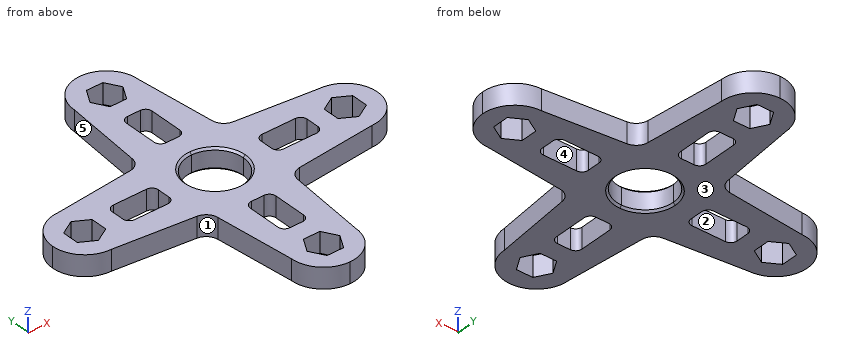
from build123d import *

# Parameters (mm, degrees)
F1_DEPTH = 8
F3_COUNT = 4
F4_R     = 5
F5_SIZE  = 0.762


with BuildPart() as f1:
    # F0 (on Top) → F1 (new body)
    with BuildSketch(Plane.XY):
        with BuildLine():
            ThreePointArc((0, 63.3), (-8.8388347648, 59.6388347648), (-12.5, 50.8))
            Line((-12.5, 50.8), (-6.4172713361, 50.8))
            Line((-6.4172713361, 50.8), (-3.208635668, 56.35752))
            Line((-3.208635668, 56.35752), (0, 56.35752))
            Line((0, 56.35752), (0, 63.3))
        make_face()
        with BuildLine():
            Line((6.4172713361, 50.8), (12.5, 50.8))
            ThreePointArc((12.5, 50.8), (8.8388347648, 59.6388347648), (0, 63.3))
            Line((0, 63.3), (0, 56.35752))
            Line((0, 56.35752), (3.208635668, 56.35752))
            Line((3.208635668, 56.35752), (6.4172713361, 50.8))
        make_face()
        with BuildLine():
            ThreePointArc((0, 38.3), (8.8388347648, 41.9611652352), (12.5, 50.8))
            Line((12.5, 50.8), (6.4172713361, 50.8))
            Line((6.4172713361, 50.8), (3.208635668, 45.24248))
            Line((3.208635668, 45.24248), (0, 45.24248))
            Line((0, 45.24248), (0, 38.3))
        make_face()
        with BuildLine():
            Line((-6.4172713361, 50.8), (-12.5, 50.8))
            ThreePointArc((-12.5, 50.8), (-8.8388347648, 41.9611652352), (0, 38.3))
            Line((0, 38.3), (0, 45.24248))
            Line((0, 45.24248), (-3.208635668, 45.24248))
            Line((-3.208635668, 45.24248), (-6.4172713361, 50.8))
        make_face()
        with BuildLine():
            ThreePointArc((-17.4128947138, 1.7438743322), (-11.7416395615, 12.9762822259), (0, 17.5))
            Line((0, 17.5), (0, 20))
            Line((0, 20), (-2.5, 20))
            ThreePointArc((-2.5, 20), (-4.267766953, 20.732233047), (-5, 22.5))
            Line((-5, 22.5), (-5, 35.5))
            ThreePointArc((-5, 35.5), (-4.267766953, 37.267766953), (-2.5, 38))
            Line((-2.5, 38), (0, 38))
            Line((0, 38), (0, 38.3))
            ThreePointArc((0, 38.3), (-8.8388347648, 41.9611652352), (-12.5, 50.8))
            Line((-12.5, 50.8), (-17.4128947138, 1.7438743322))
        make_face()
        with BuildLine():
            Line((0, 20), (0, 17.5))
            ThreePointArc((0, 17.5), (11.7416395615, 12.9762822259), (17.4128947138, 1.7438743322))
            Line((17.4128947138, 1.7438743322), (12.5, 50.8))
            ThreePointArc((12.5, 50.8), (8.8388347648, 41.9611652352), (0, 38.3))
            Line((0, 38.3), (0, 38))
            Line((0, 38), (2.5, 38))
            ThreePointArc((2.5, 38), (4.267766953, 37.267766953), (5, 35.5))
            Line((5, 35.5), (5, 22.5))
            ThreePointArc((5, 22.5), (4.267766953, 20.732233047), (2.5, 20))
            Line((2.5, 20), (0, 20))
        make_face()
        with BuildLine():
            ThreePointArc((17.4128947138, 1.7438743322), (11.7416395615, 12.9762822259), (0, 17.5))
            ThreePointArc((0, 17.5), (-11.7416395615, 12.9762822259), (-17.4128947138, 1.7438743322))
            ThreePointArc((-17.4128947138, 1.7438743322), (-0.8730242003, -17.4782101128), (17.5, 0))
            ThreePointArc((17.5, 0), (17.4782101128, 0.8730242003), (17.4128947138, 1.7438743322))
        make_face()
        with BuildLine():
            ThreePointArc((0, 11.025), (7.7958522626, 7.7958522626), (11.025, 0))
            ThreePointArc((11.025, 0), (-7.7958522626, -7.7958522626), (0, 11.025))
        make_face(mode=Mode.SUBTRACT)
    extrude(amount=F1_DEPTH)

    # F3: F1 ×4 about axis
    f3_axis = Axis((0, 0, 24.1194125265), (0, 0, 1))


with BuildPart() as f1_1:
    add(f1.part)
    for i in range(1, F3_COUNT):
        add(f1.part.rotate(f3_axis, i * 360 / F3_COUNT))

    # F4
    f4_edges = [f1_1.edges().sort_by_distance(p)[0] for p in [
        (15.986516, 15.986516, 4),
        (-15.986516, 15.986516, 4),
        (-15.986516, -15.986516, 4),
        (15.986516, -15.986516, 4),
    ]]
    fillet(f4_edges, radius=F4_R)

    # F5
    f5_edges = [f1_1.edges().sort_by_distance(p)[0] for p in [
        (0, -11.025, 8),
        (0, -11.025, 0),
    ]]
    chamfer(f5_edges, length=F5_SIZE)


solid = f1_1.part
Part model, mm, in its own coordinate system. Face numbers are marked on the shaded views. A direction names the side the tool comes from. Give positions to 0.01 mm unless a question says otherwise; leave off trailing zeros. Loops run counter-clockwise (first coordinate to the right, second up) from the corner with the lowest first, then second, coordinate; pieces in that order, holes last. Notation, with made-up numbers: (49, 8.25) -> (102, 8.25) arc R33 ccw to (102, 43.25) -> close; hole circle Ø4 at (30, 37.25). An arc over 180 degrees is marked (long way). Write each question's results on one line, items separated by ' | '. Start each with the question number.
Q1. Band-saw the part on B-B on z = 5.25. Count the separate pieces of the cut face and the enclosed holes in it, plus the area to 3 significant figures.
Q2. Band-saw the part on A-A on x = -28. List the corners of the cut face in (y, z), plus the area to 3 significant figures.
Q3. Pull direction X, two halves, no side cores. Call the marked faces 1, 2 and 3: +X half, -X half, draft (parallel to the pull), parting line (faces both ways), or undercut.
Q4. Pin check, flat tips, straight feed: P1, Ø4, axis at x = 44.5, z = 4, coming from the +Y side; P2, Ø4, axis at y = 29, z = 4.5, coming from the -X side; P3, Ø4, axis at x = 28, z = 5, coming from the -Y side. Stop position of each tip, or through.
Q5. Wall check: L1, parallel to Y at x = 4.5, z = 2.5; L2, parallel to X at y = 33.5, z = 5.5; L3, parallel to X at y = -46.5, z = 4. Give the ranges that are in metal, low to high.
Q6. Which spindle directions (+Z, -Z, +X, -X, +Y, -Y) get a long thin tool onto all of the face, cutting with end or side? Do the marked faces 4 and 5. Say none if no direction does.
Results are:
1) separate pieces: 1 | enclosed holes: 9 | area: 4,480 mm²
2) outline: (-14.78, 0) -> (-5, 0) -> (-5, 8) -> (-14.78, 8) -> close; (5, 0) -> (14.78, 0) -> (14.78, 8) -> (5, 8) -> close | area: 157 mm²
3) face 1: -X half | face 2: undercut | face 3: draft
4) P1: stops at y = 13.33 | P2: stops at x = -14.88 | P3: stops at y = -14.98
5) L1: y = -62.46 to -54.12, -47.48 to -37, -21 to -10.06, 10.06 to 21, 37 to 47.48, 54.12 to 62.46 | L2: x = -14.23 to -5, 5 to 14.23 | L3: x = -12.93 to -3.93, 3.93 to 12.93
6) face 4: +Z, -Z | face 5: +Z, -Z, -X, +Y
